from build123d import *

# Parameters (mm, degrees)
BOSS_EXTRUDE1_DEPTH = 1
SKETCH2_R           = 0.675
BOSS_EXTRUDE2_DEPTH = 5
SKETCH3_R           = 0.675
BOSS_EXTRUDE3_DEPTH = 4


with BuildPart() as part:
    # Sketch1 → Boss-Extrude1 (new, symmetric)
    with BuildSketch(Plane(origin=(0, 0, 0), x_dir=(0, 0, -1), z_dir=(1, 0, 0))):
        with BuildLine():
            Line((-2.5, 1.5), (2.5, 1.5))
            ThreePointArc((2.5, 1.5), (4, 0), (2.5, -1.5))
            Line((2.5, -1.5), (-2.5, -1.5))
            ThreePointArc((-2.5, -1.5), (-4, 0), (-2.5, 1.5))
        make_face()
    extrude(amount=BOSS_EXTRUDE1_DEPTH, both=True)

    # Sketch2 → Boss-Extrude2 (add)
    with BuildSketch(Plane(origin=(0, 0, 0), x_dir=(0, 0, -1), z_dir=(1, 0, 0))):
        with Locations((-2.5, 0)):
            Circle(SKETCH2_R)
    extrude(amount=BOSS_EXTRUDE2_DEPTH)

    # Sketch3 → Boss-Extrude3 (add)
    with BuildSketch(Plane(origin=(0, 0, 0), x_dir=(0, 0, -1), z_dir=(1, 0, 0))):
        with Locations((2.5, 0)):
            Circle(SKETCH3_R)
    extrude(amount=BOSS_EXTRUDE3_DEPTH)


solid = part.part
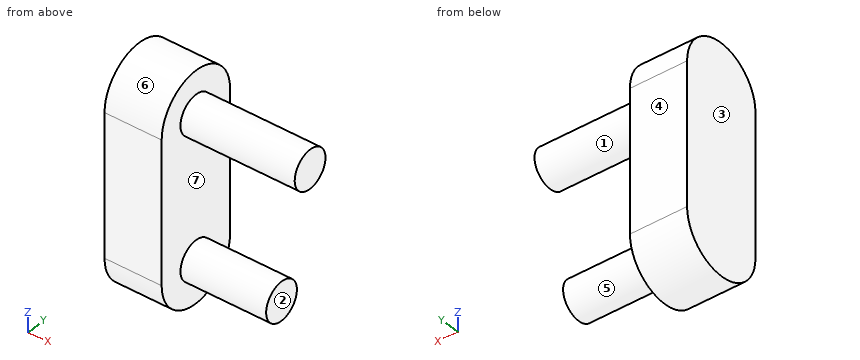
Source: CAD feature listing. Evaluate the final solid. Frame: model axes, mm. Face numbers are marked on the shaded views. A direction names the side the tool comes from. Coordinates: 2 decimals unless noted, no trailing zeros. Loops run counter-clockwise (first coordinate to the right, second up) from the corner with the lowest first, then second, coordinate; pieces in that order, holes last. Notation, with made-up numbers: (4, -32.75) - (14, -32.75) arc R8 cw to (14, -19.75) - close; hole circle Ø10 at (71, 1). An arc over 180 degrees is marked (long way). One line per question, with ' | ' between items.
1) Set-up query: the marked faces 1, 2 and 3. Return all of +Z, -Z, +X, -X, +Y, -Y with unobstructed straight access to the full face (end or side cutting, diameter ignored); none if empty.
Report:
face 1: +X | face 2: -Z, +X, +Y, -Y | face 3: +Z, -Z, -X, +Y, -Y
2) Section B-B, the plane x = 2.3. Return loops of the section in (y, z) (3 decimals).
Report:
outline: circle Ø1.35 at (0, -2.5); circle Ø1.35 at (0, 2.5)
3) Pull-direction query (Z, two-part tool) for the marked faces 4, 5, 6 and 7; classes: released by +Z, released by -Z, zero draft, split by the parting line, or undercut.
Report:
face 4: zero draft | face 5: undercut | face 6: released by +Z | face 7: undercut
4) Line query: line 1 along X through (y, z) = (0.6, -2.5); line 2 along X through (y, z) = (1.45, -2); line 3 along Z through (x, y) = (3.75, 0.05). Output: solid intervals per line, ascending.
Report:
line 1: x = -1 to 4 | line 2: x = -1 to 1 | line 3: z = -3.17 to -1.83, 1.83 to 3.17
5) First-contact query: P1, Ø1, axis at x = 1, y = -1, coming from the +Z side. Flat tip, straight axial feed; report the tip coordinate or a pass-through.
Report:
P1: stops at z = 3.91
6) Section A-A, the plane y = 0. Return loops of the section in (x, z) (3 decimals), then the cut area to 4 significant figures.
Report:
outline: (-1, -4) - (1, -4) - (1, -3.175) - (4, -3.175) - (4, -1.825) - (1, -1.825) - (1, 1.825) - (5, 1.825) - (5, 3.175) - (1, 3.175) - (1, 4) - (-1, 4) - close | area: 25.45 mm²
7) Section D-D, the plane z = -0.25. Return loops of the section in (x, y).
Report:
outline: (-1, -1.5) - (1, -1.5) - (1, 1.5) - (-1, 1.5) - close
8) Section C-C, the plane x = 4.5. Return loops of the section in (y, z) (3 decimals), then the cut area to 3 significant figures.
Report:
outline: circle Ø1.35 at (0, 2.5) | area: 1.43 mm²
